Here's how the part is built. I have some questions about the finished solid (model axes, mm). A direction names the side the tool comes from. Coordinates: 2 decimals unless noted, no trailing zeros. Loops run counter-clockwise (first coordinate to the right, second up) from the corner with the lowest first, then second, coordinate; pieces in that order, holes last. Notation, with made-up numbers: (-22.75, -14) -> (10.25, -14) arc R18 ccw to (10.25, -9) -> close; hole circle Ø1 at (-15.75, 55.5). An arc over 180 degrees is marked (long way). Answer as a JSON object with one key per item and string values. Group by question number.
Q1. Thinking about a two-plate mould opening in Z: for faces 4 (the cylindrical face through (33.35, 99.99, 35.875)), 5 (the flat face through (3.175, 51, 20)), 6 (the flat face through (53, 2, 0)), which applies, released by +Z, released by -Z, zero draft, split by the parting line, or undercut?
Q2. I want a section at B-B on y = 61.5. Write out the boundary of the cut face in (x, z) (3 decimals), then the cut area to 3 significant figures.
Q3. I want a section at D-D on z = 25. Write out the boundary of the cut face in (x, y) (3 decimals).
Q4. I want a section at A-A on x = 114. Write out the boundary of the cut face in (y, z) (3 decimals).
Q5. I'm going to push a flat-ended pin straight in: pin 1 (10.5 mm diameter, centred on x = 31.2, z = 7.5, fed in from -Y). Where does the tip first touch, or does it pass through?
Q6. On a 3-axis mill with a long thin cutter (end or side, diameter ignored), from which of +Z, -Z, +X, -X, +Y, -Y can I reach the whole of each face in a straight line? I mean faces 1 (the flat face through (75, 3.175, 20)), 2 (the cylindrical face through (117.204, 99.99, 7.678)), 3 (the flat face through (152.4, 50, 20)). Say none if no direction works.
Q7. I need wall thicknesses on line 1 (Z direction, x = 31.2, y = 99.5) (1 decimal); line 2 (Y direction, x = 54.5, z = 8) (3 decimals); line 3 (X direction, y = 79, z = 34) (3 decimals). Which ranges of each line are inside material? Lowest first, please.
Q8. I want a section at C-C on x = 31.2. Write out the boundary of the cut face in (y, z) (1 decimal).
Autodesk Inventor part; units mm, degrees
ref_plane "YZ Plane" through (0, 0, 0) normal (1, 0, 0) x (0, 1, 0)
ref_plane "XZ Plane" through (0, 0, 0) normal (0, 1, 0) x (-1, 0, 0)
ref_plane "XY Plane" through (0, 0, 0) normal (0, 0, 1) x (1, 0, 0)
sketch "Sketch1" plane through (0, 0, 0) normal (0, 0, 1) x (1, 0, 0)
  line L0 (0, 0) -> (152.4, 0)
  line L1 (152.4, 0) -> (152.4, 101.6)
  line L2 (152.4, 101.6) -> (0, 101.6)
  line L3 (0, 101.6) -> (0, 0)
  dimension "d0" = 152.4
  dimension "d1" = 101.6
extrude "Extrusion1" add sketch "Sketch1" along normal blind 40.005
shell "Shell1" thickness 3.175 removed faces 2 at (50.8, 67.7333, 0) at (50.8, 67.7333, 40.005)
sketch "Sketch2" plane through (3.175, 98.425, 0) normal (0, -1, 0) x (1, 0, 0)
  circle A0 centre (118.025, 7.5025) radius 4
  circle A1 centre (28.025, 7.5025) radius 4
  line L0 (-3.175, 0) -> (-3.175, 40.005) construction
  line L1 (-3.175, 0) -> (149.225, 0) construction
  circle A2 centre (118.025, 32.5025) radius 4
  circle A3 centre (28.025, 32.5025) radius 4
  line L2 (118.025, 7.5025) -> (28.025, 7.5025) construction
  line L3 (28.025, 7.5025) -> (28.025, 32.5025)
  line L4 (28.025, 32.5025) -> (118.025, 32.5025) construction
  line L5 (118.025, 32.5025) -> (118.025, 7.5025) construction
  point P0 (73.025, 7.5025)
  point P1 (73.025, 0)
  point P2 (28.025, 20.0025)
  point P3 (-3.175, 20.0025)
  dimension "d5" = 8
  dimension "d6" = 25
  dimension "d7" = 90
extrude "Extrusion2" cut sketch "Sketch2" against normal up to surface (3.175 mm away)
properties part number "YGANTRYTUBE"
Result set:
{
 "1": {"face 4": "undercut", "face 5": "zero draft", "face 6": "released by -Z"},
 "2": {"outline": "(0, 0) -> (3.175, 0) -> (3.175, 40.005) -> (0, 40.005) -> close; (149.225, 0) -> (152.4, 0) -> (152.4, 40.005) -> (149.225, 40.005) -> close", "area": "254 mm²"},
 "3": {"outline": "(0, 0) -> (152.4, 0) -> (152.4, 101.6) -> (0, 101.6) -> close; hole (3.175, 3.175) -> (149.225, 3.175) -> (149.225, 98.425) -> (3.175, 98.425) -> close"},
 "4": {"outline": "(0, 0) -> (3.175, 0) -> (3.175, 40.005) -> (0, 40.005) -> close; (98.425, 0) -> (101.6, 0) -> (101.6, 40.005) -> (98.425, 40.005) -> close"},
 "5": {"pin 1": "stops at y = 0"},
 "6": {"face 1": "+Z, -Z", "face 2": "+Y", "face 3": "+Z, -Z, +X, +Y, -Y"},
 "7": {"line 1": "z = 0 to 3.5, 11.5 to 28.5, 36.5 to 40", "line 2": "y = 0 to 3.175, 98.425 to 101.6", "line 3": "x = 0 to 3.175, 149.225 to 152.4"},
 "8": {"outline": "(0, 0) -> (3.2, 0) -> (3.2, 40) -> (0, 40) -> close; (98.4, 0) -> (101.6, 0) -> (101.6, 3.5) -> (98.4, 3.5) -> close; (98.4, 11.5) -> (101.6, 11.5) -> (101.6, 28.5) -> (98.4, 28.5) -> close; (98.4, 36.5) -> (101.6, 36.5) -> (101.6, 40) -> (98.4, 40) -> close"}
}
